```python
from build123d import *

# Parameters (mm, degrees)
BOSS_EXTRUDE1_DEPTH                   = 3
TAP_DRILL_FOR_M4X0_7_TAP1_D           = 3.3
TAP_DRILL_FOR_M4X0_7_TAP1_CSINK_D     = 3.35
TAP_DRILL_FOR_M4X0_7_TAP1_CSINK_ANGLE = 90
CIRPATTERN1_COUNT                     = 4
SKETCH11_W                            = 60
SKETCH11_H                            = 5.997041234
BOSS_EXTRUDE2_DEPTH                   = 22
CUT_EXTRUDE4_DEPTH                    = 35
CHAMFER1_SIZE                         = 3
CHAMFER2_SIZE                         = 3


with BuildPart() as part:
    # Sketch1 → Boss-Extrude1 (new body)
    with BuildSketch(Plane.XY):
        with BuildLine():
            Line((-16.785410333, -38.37), (-3.5, -38.37))
            add(Edge.make_bspline(
                [(-3.5, -38.37), (-2.487663845, -38.37), (-1.180873463, -37.25254604), (-1.493022396, -34.741636396), (0, -34.57)],
                knots=[0, 0, 0, 0, 0.364574194, 1, 1, 1, 1], degree=3))
            add(Edge.make_bspline(
                [(3.5, -38.37), (2.522461063, -38.37), (1.117320535, -37.441425493), (1.462124558, -34.862224896), (0, -34.57)],
                knots=[0, 0, 0, 0, 0.352042618, 1, 1, 1, 1], degree=3))
            Line((3.5, -38.37), (16.785410333, -38.37))
            ThreePointArc((16.785410333, -38.37), (41.88086556, 0), (16.785410333, 38.37))
            Line((16.785410333, 38.37), (3.5, 38.37))
            add(Edge.make_bspline(
                [(3.5, 38.37), (2.522461063, 38.37), (1.117320535, 37.441425493), (1.462124558, 34.862224896), (0, 34.57)],
                knots=[0, 0, 0, 0, 0.352042618, 1, 1, 1, 1], degree=3))
            add(Edge.make_bspline(
                [(-3.5, 38.37), (-2.487663845, 38.37), (-1.180873463, 37.25254604), (-1.493022396, 34.741636396), (0, 34.57)],
                knots=[0, 0, 0, 0, 0.364574194, 1, 1, 1, 1], degree=3))
            Line((-3.5, 38.37), (-16.785410333, 38.37))
            ThreePointArc((-16.785410333, 38.37), (-41.88086556, 0), (-16.785410333, -38.37))
        make_face()
        with BuildLine():
            Line((11.497282288, -15.75), (-11.497282288, -15.75))
            ThreePointArc((-11.497282288, -15.75), (-19.5, 0), (-11.497282288, 15.75))
            Line((-11.497282288, 15.75), (11.497282288, 15.75))
            ThreePointArc((11.497282288, 15.75), (19.5, 0), (11.497282288, -15.75))
        make_face(mode=Mode.SUBTRACT)
    extrude(amount=BOSS_EXTRUDE1_DEPTH)

    # Tap Drill for M4x0.7 Tap1 (through all)
    with Locations(Plane(origin=(0, 32, 0), x_dir=(-1, 0, 0), z_dir=(0, 0, -1))):
        with Locations((0, 0)):
            tap_drill_for_m4x0_7_tap1 = CounterSinkHole(TAP_DRILL_FOR_M4X0_7_TAP1_D / 2, TAP_DRILL_FOR_M4X0_7_TAP1_CSINK_D / 2, counter_sink_angle=TAP_DRILL_FOR_M4X0_7_TAP1_CSINK_ANGLE)

    # CirPattern1: Tap Drill for M4x0.7 Tap1 ×4 about axis
    cirpattern1_axis = Axis((0, 0, 0), (0, 0, 1))
    for i in range(1, CIRPATTERN1_COUNT):
        add(tap_drill_for_m4x0_7_tap1.rotate(cirpattern1_axis, i * 360 / CIRPATTERN1_COUNT), mode=Mode.SUBTRACT)

    # Sketch11 → Boss-Extrude2 (add, symmetric)
    with BuildSketch(Plane(origin=(0, 0, 0), x_dir=(0, 0, -1), z_dir=(1, 0, 0))):
        with Locations((-33, 18.748520617)):
            Rectangle(SKETCH11_W, SKETCH11_H)
        with Locations((-33, -18.748520617)):
            Rectangle(SKETCH11_W, SKETCH11_H)
    extrude(amount=BOSS_EXTRUDE2_DEPTH, both=True)

    # Sketch9 → Cut-Extrude4 (cut, symmetric)
    with BuildSketch(Plane(origin=(28, 0, 0), x_dir=(0, 0, -1), z_dir=(0, -1, 0))):
        with BuildLine():
            Line((-19.7, -13.5), (-31, -13.5))
            ThreePointArc((-31, -13.5), (-32.5, -15), (-31, -16.5))
            Line((-31, -16.5), (-19.7, -16.5))
            ThreePointArc((-19.7, -16.5), (-18.2, -15), (-19.7, -13.5))
        make_face()
        with BuildLine():
            Line((-19.7, -39.5), (-31, -39.5))
            ThreePointArc((-31, -39.5), (-32.5, -41), (-31, -42.5))
            Line((-31, -42.5), (-19.7, -42.5))
            ThreePointArc((-19.7, -42.5), (-18.2, -41), (-19.7, -39.5))
        make_face()
    extrude(amount=CUT_EXTRUDE4_DEPTH, both=True, mode=Mode.SUBTRACT)

    # Chamfer1
    chamfer1_edges = [part.edges().sort_by_distance(p)[0] for p in [
        (0, 21.747041234, 3),
    ]]
    chamfer(chamfer1_edges, length=CHAMFER1_SIZE)

    # Chamfer2
    chamfer2_edges = [part.edges().sort_by_distance(p)[0] for p in [
        (0, -21.747041234, 3),
    ]]
    chamfer(chamfer2_edges, length=CHAMFER2_SIZE)


solid = part.part
```
Input: part model. Units: mm. Frame: model coordinates. A direction names the side the tool comes from. Round coordinates to 2 decimals unless told otherwise and drop trailing zeros. Loops run counter-clockwise (first coordinate to the right, second up) from the corner with the lowest first, then second, coordinate; pieces in that order, holes last.
1) Pull-direction query (X, two-part tool) for faces 1 (the cylindrical face through (13, -18.7, 32.5)), 2 (the flat face through (-22, 18, 33)), 3 (the flat face through (-19, 9, 3)); classes: released by +X, released by -X, zero draft, split by the parting line, or undercut.
Ans:
face 1: undercut
face 2: released by -X
face 3: zero draft
2) Set-up query: faces 4 (the flat face through (22, -18, 33)), 5 (the flat face through (10, 38.37, 1)), 6 (the flat face through (-14.5, -19, 25)). Return all of +Z, -Z, +X, -X, +Y, -Y with unobstructed straight access to the full face (end or side cutting, diameter ignored); none if empty.
Ans:
face 4: +Z, +X, +Y, -Y
face 5: +Z, -Z, +X, -X, +Y
face 6: +Y, -Y
3) Pin query (flat end, axial travel): pin 1 (3 mm diameter, centred on y = -18, z = 23.5, fed in from +X); pin 2 (5 mm diameter, centred on y = -20, z = 27.5, fed in from -X); pin 3 (22 mm diameter, centred on x = 1.5, z = 35, fed in from +Y); pin 4 (3 mm diameter, centred on x = 32, y = 0, fed in from +Z). Return the tip coordinate at first contact, or that it passes through.
Ans:
pin 1: stops at x = 22
pin 2: stops at x = -22
pin 3: stops at y = 21.75
pin 4: passes through
4) Material intervals for line 1 (X direction, y = -21, z = 29); line 2 (Y direction, x = -13, z = 43); line 3 (Z direction, x = 27.5, y = -24.5), sorted ascending.
Ans:
line 1: x = -22 to -14.5, -11.5 to 11.5, 14.5 to 22
line 2: y = -21.75 to -15.75, 15.75 to 21.75
line 3: z = 0 to 3
5) Section query C-C on x = 9.5. Return the cut outline in (y, z), plus the area to 3 significant figures.
Ans:
outline: (-38.37, 0) - (-15.75, 0) - (-15.75, 63) - (-21.75, 63) - (-21.75, 6) - (-24.75, 3) - (-38.37, 3) - close; (15.75, 0) - (38.37, 0) - (38.37, 3) - (24.75, 3) - (21.75, 6) - (21.75, 63) - (15.75, 63) - close
area: 864 mm2
6) Section query A-A on z = 47. Return the cut outline in (x, y), plus the area to 3 significant figures.
Ans:
outline: (-22, -21.75) - (22, -21.75) - (22, -15.75) - (-22, -15.75) - close; (-22, 15.75) - (22, 15.75) - (22, 21.75) - (-22, 21.75) - close
area: 528 mm2
7) Section query D-D on z = 23.5. Return the cut outline in (x, y), plus the area to 3 significant figures.
Ans:
outline: (-22, -21.75) - (-14.5, -21.75) - (-14.5, -15.75) - (-22, -15.75) - close; (-22, 15.75) - (-14.5, 15.75) - (-14.5, 21.75) - (-22, 21.75) - close; (-11.5, -21.75) - (11.5, -21.75) - (11.5, -15.75) - (-11.5, -15.75) - close; (-11.5, 15.75) - (11.5, 15.75) - (11.5, 21.75) - (-11.5, 21.75) - close; (14.5, -21.75) - (22, -21.75) - (22, -15.75) - (14.5, -15.75) - close; (14.5, 15.75) - (22, 15.75) - (22, 21.75) - (14.5, 21.75) - close
area: 456 mm2
8) Section query B-B on y = 0. Return the cut outline in (x, z) (3 decimals), plus the area to 3 significant figures.
Ans:
outline: (-41.881, 0) - (-33.675, 0) - (-33.65, 0.025) - (-33.65, 3) - (-41.881, 3) - close; (-30.35, 0.025) - (-30.325, 0) - (-19.5, 0) - (-19.5, 3) - (-30.35, 3) - close; (19.5, 0) - (30.325, 0) - (30.35, 0.025) - (30.35, 3) - (19.5, 3) - close; (33.65, 0.025) - (33.675, 0) - (41.881, 0) - (41.881, 3) - (33.65, 3) - close
area: 114 mm2
